Geometry check sheet. Reference: drawing and pictorial views, mm from the part's lowest x, y, z. Round coordinates to 2 decimals unless told otherwise and drop trailing zeros. Write each loop counter-clockwise with the first axis right and the second up, starting at its lowest first coordinate (ties: lowest second). Pieces come first, ordered by that corner, then holes. Notation, with made-up numbers: (78, 68) -> (110, 68) arc R27 ccw to (110, 98) -> close; hole circle Ø9 at (44, -35.75). An arc over 180 degrees is marked (long way). Answer as a JSON object with one key per item and string values. Group by question number.
(1) Gauge pin test, flat end, axial feed: pin 1 Ø1 at (y, z) = (1, 14) entering from -X (1 decimal). Record the tip position at first contact, or that the pin passes through.
(2) Sectioned sample at B-B on z = 12.5. Record the cut outline in (x, y) (1 decimal).
(3) Scan lines: L1, parallel to X at y = 0.45, z = 9.5 (1 decimal); L2, parallel to Z at x = 23.5, y = 0.75; L3, parallel to Z at x = 7.5, y = 1.65. Record each from-to range of solid material in increasing order. Write a range as from..to.
(4) Sectioned sample at C-C on x = 8.5. Record the cut outline in (y, z).
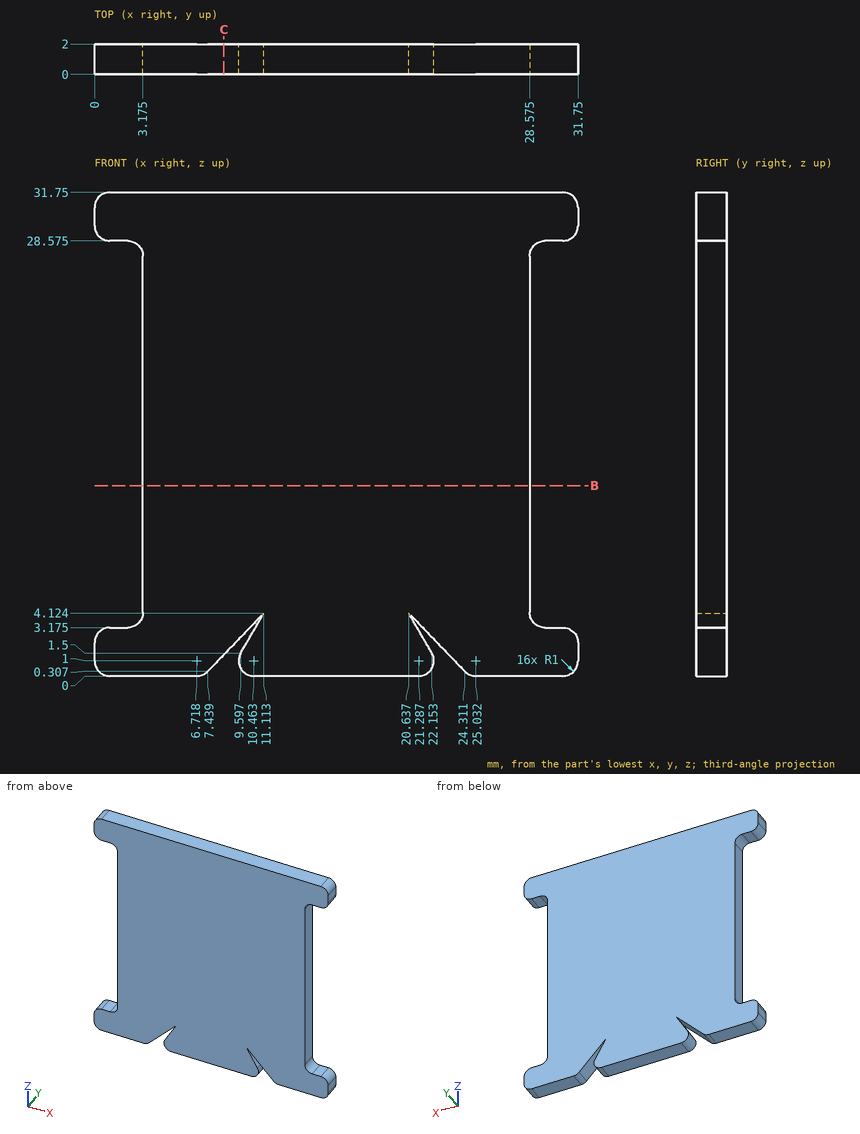
Computed values:
{
 "1": {"pin 1": "x = 3.2"},
 "2": {"outline": "(3.2, 0) -> (28.6, 0) -> (28.6, 2) -> (3.2, 2) -> close"},
 "3": {"L1": "3.2..28.6", "L2": "1.15..31.75", "L3": "0.37..31.75"},
 "4": {"outline": "(0, 1.41) -> (2, 1.41) -> (2, 31.75) -> (0, 31.75) -> close"}
}
